Here's how the part is built. I have some questions about the finished solid (model axes, mm). Face numbers are marked on the shaded views. A direction names the side the tool comes from. Coordinates: 2 decimals unless noted, no trailing zeros. Write each loop counter-clockwise with the first axis right and the second up, starting at its lowest first coordinate (ties: lowest second). Pieces come first, ordered by that corner, then holes. Notation, with made-up numbers: (-29, 62) -> (-13, 62) arc R9 cw to (-13, 72) -> close; hole circle Ø4 at (86.25, 76). An arc over 180 degrees is marked (long way). Use a Markdown table: item, result. Add a question column.
Item 1: On a 3-axis mill with a long thin cutter (end or side, diameter ignored), from which of +Z, -Z, +X, -X, +Y, -Y can I reach the whole of each face in a straight line? I mean the marked faces 4 and 5. Say none if no direction works.
Item 2: Imagine slicing it at C-C, the plane x = 0. Write out the boundary of the cut face in (y, z).
Item 3: Will these pins go through, and if not, where does the flat tip stop? pin 1 Ø6 at (x, z) = (-0.5, 15.5) entering from +Y; pin 2 Ø7.5 at (x, z) = (0, 12.7) entering from +Y; pin 3 Ø4 at (x, y) = (-8.5, 3.5) entering from +Z.
Item 4: If we mould it in two halves opening along Y, with no side actions, what happens to the marked faces 1, 2 and 3? For each: pulls with the +Y half, pulls with the -Y half, needs draft (parallel to the pull), parting line crosses it, or undercut.
Item 5: If I drill on line 1 along X through (y, z) = (20, 21.25); line 2 along Z through (x, y) = (0, -1); line 3 along Z through (x, y) = (0, -3), over which ranges is the centre line in solid material (lowest first)? Write a range as from..to.
Item 6: Imagine slicing it at D-D, the plane z = 2.5. Write out the boundary of the cut face in (x, y), and give its area (3 significant figures).
Item 7: Imagine slicing it at B-B, the plane z = 12.7. Write out the boundary of the cut face in (x, y).
Item 8: Imagine slicing it at A-A, the plane y = 7.5. Write out the boundary of the cut face in (x, z), and give its area (3 significant figures).
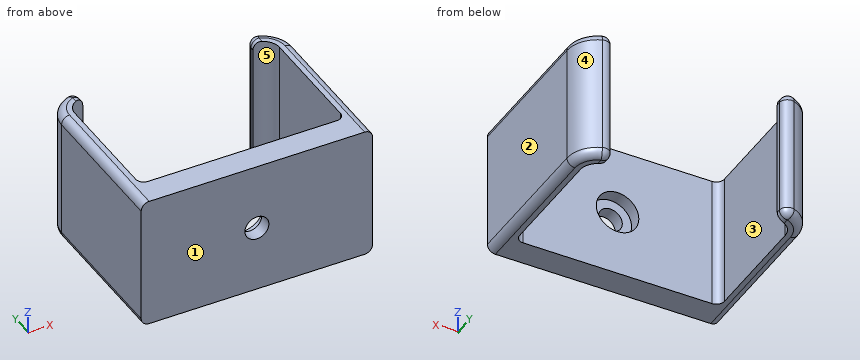
```python
from build123d import *

# Parameters (mm, degrees)
F1_DEPTH = 25.4
F2_R     = 2.286
F3_DEPTH = 5.08
F4_R     = 4.064
F5_DEPTH = 2.54
F6_R     = 1.524


with BuildPart() as f1:
    # F0 (on Top) → F1 (new body)
    with BuildSketch(Plane.XY):
        with BuildLine():
            ThreePointArc((-16.256, 28.702), (-20.386918, 26.990918), (-22.098, 22.86))
            Line((-22.098, 22.86), (-22.098, -5.08))
            Line((-22.098, -5.08), (22.098, -5.08))
            Line((22.098, -5.08), (22.098, 22.86))
            ThreePointArc((22.098, 22.86), (20.386918, 26.990918), (16.256, 28.702))
            Line((16.256, 28.702), (16.256, 26.162))
            ThreePointArc((16.256, 26.162), (18.590867, 25.194867), (19.558, 22.86))
            Line((19.558, 22.86), (19.558, 0))
            Line((19.558, 0), (-19.558, 0))
            Line((-19.558, 0), (-19.558, 22.86))
            ThreePointArc((-19.558, 22.86), (-18.590867, 25.194867), (-16.256, 26.162))
            Line((-16.256, 26.162), (-16.256, 28.702))
        make_face()
    extrude(amount=F1_DEPTH)

    # F2 (on face) → F3 (cut, through all)
    with BuildSketch(Plane.XZ.offset(5.08)):
        with Locations((0, 12.7)):
            Circle(F2_R)
    extrude(amount=-F3_DEPTH, mode=Mode.SUBTRACT)

    # F4 (on face) → F5 (cut)
    with BuildSketch(Plane(origin=(0, 0, 0), x_dir=(-1, 0, 0), z_dir=(0, 1, 0))):
        with Locations((0, 12.7)):
            Circle(F4_R)
    extrude(amount=-F5_DEPTH, mode=Mode.SUBTRACT)

    # F6
    f6_edges = [f1.edges().sort_by_distance(p)[0] for p in [
        (-20.386918, 26.990918, 25.4),
        (20.386918, 26.990918, 25.4),
        (20.386918, 26.990918, 0),
        (-22.098, 8.89, 0),
        (-19.558, 0, 12.7),
        (19.558, 0, 12.7),
        (-16.256, 28.702, 12.7),
        (16.256, 28.702, 12.7),
        (-16.256, 27.432, 25.4),
        (16.256, 27.432, 25.4),
        (16.256, 27.432, 0),
        (-16.256, 27.432, 0),
    ]]
    fillet(f6_edges, radius=F6_R)


solid = f1.part
```
Ans:
| question | item | result |
|---|---|---|
| 1 | face 4 | +Z, -Z, +X, +Y |
| 1 | face 5 | +Z, -Z |
| 2 | outline | (-5.08, 0) -> (0, 0) -> (0, 8.64) -> (-2.54, 8.64) -> (-2.54, 10.41) -> (-5.08, 10.41) -> close; (-5.08, 14.99) -> (-2.54, 14.99) -> (-2.54, 16.76) -> (0, 16.76) -> (0, 25.4) -> (-5.08, 25.4) -> close |
| 3 | pin 1 | stops at y = 0 |
| 3 | pin 2 | stops at y = -2.54 |
| 3 | pin 3 | passes through |
| 4 | face 1 | pulls with the -Y half |
| 4 | face 2 | needs draft |
| 4 | face 3 | undercut |
| 5 | line 1 | x = -22.1..-19.56, 19.56..22.1 |
| 5 | line 2 | z = 0..8.64, 16.76..25.4 |
| 5 | line 3 | z = 0..10.41, 14.99..25.4 |
| 6 | outline | (-22.1, -5.08) -> (22.1, -5.08) -> (22.1, 22.86) arc R5.84 ccw to (18.32, 28.33) arc R1.52 ccw to (16.26, 26.9) -> (16.26, 26.16) arc R3.3 cw to (19.56, 22.86) -> (19.56, 1.52) arc R1.52 cw to (18.03, 0) -> (-18.03, 0) arc R1.52 cw to (-19.56, 1.52) -> (-19.56, 22.86) arc R3.3 cw to (-16.26, 26.16) -> (-16.26, 26.9) arc R1.52 ccw to (-18.32, 28.33) arc R5.84 ccw to (-22.1, 22.86) -> close |
| 6 | area | 376 mm^2 |
| 7 | outline | (-22.1, -5.08) -> (-2.29, -5.08) -> (-2.29, -2.54) -> (-4.06, -2.54) -> (-4.06, 0) -> (-18.03, 0) arc R1.52 cw to (-19.56, 1.52) -> (-19.56, 22.86) arc R3.3 cw to (-16.26, 26.16) -> (-16.26, 26.9) arc R1.52 ccw to (-18.32, 28.33) arc R5.84 ccw to (-22.1, 22.86) -> close; (2.29, -5.08) -> (22.1, -5.08) -> (22.1, 22.86) arc R5.84 ccw to (18.32, 28.33) arc R1.52 ccw to (16.26, 26.9) -> (16.26, 26.16) arc R3.3 cw to (19.56, 22.86) -> (19.56, 1.52) arc R1.52 cw to (18.03, 0) -> (4.06, 0) -> (4.06, -2.54) -> (2.29, -2.54) -> close |
| 8 | outline | (-22.1, 1.52) arc R1.52 ccw to (-20.57, 0) -> (-19.56, 0) -> (-19.56, 25.4) -> (-20.57, 25.4) arc R1.52 ccw to (-22.1, 23.88) -> close; (19.56, 0) -> (20.57, 0) arc R1.52 ccw to (22.1, 1.52) -> (22.1, 23.88) arc R1.52 ccw to (20.57, 25.4) -> (19.56, 25.4) -> close |
| 8 | area | 127 mm^2 |
